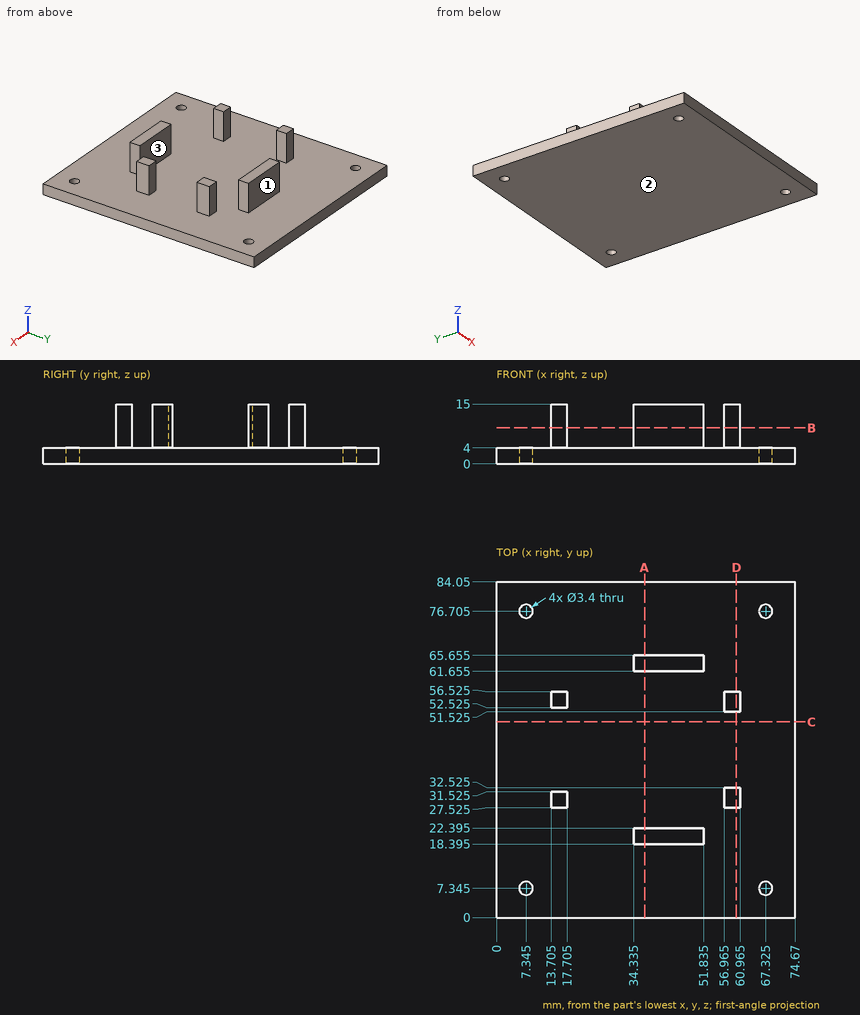
Geometry: see drawing. Coordinates: mm, zero at the bounding-box minimum. A direction names the side the tool comes from. Round coordinates to 2 decimals unless told otherwise and drop trailing zeros. Order: outer loops, then holes, each group sorted by start corner. A loop starts at its lowest first (then second) coordinate and runs counter-clockwise, first axis right, second up. Notation, with made-up numbers: (66.5, 57.25) -> (118.5, 57.25) arc R23 cw to (118.5, 86.25) -> close; hole circle Ø1 at (-29.5, 41). An arc over 180 degrees is marked (long way). Answer as CSV lines item,"result".
Item 1: Section A-A, the plane x = 37. Return loops of the section in (y, z) (3 decimals), plus the area to 3 significant figures.
A:
outline,"(0, 0) -> (84.05, 0) -> (84.05, 4) -> (65.655, 4) -> (65.655, 15) -> (61.655, 15) -> (61.655, 4) -> (22.395, 4) -> (22.395, 15) -> (18.395, 15) -> (18.395, 4) -> (0, 4) -> close"
area,"424 mm²"
Item 2: Reachability of the marked faces 1, 2 and 3 from +Z, -Z, +X, -X, +Y, -Y: full face, straight path, thin tool, end or side. Return the list, or none.
A:
face 1,"+Z, +X, -X, +Y"
face 2,"-Z, +X, -X, +Y, -Y"
face 3,"+Z, +X, -X"
Item 3: Pin query (flat end, axial travel): pin 1 Ø4.5 at (y, z) = (20.5, 10) entering from +X (3 decimals); pin 2 Ø3 at (x, z) = (15, 8.5) entering from -Y (3 decimals); pin 3 Ø3 at (x, z) = (50, 8.5) entering from -Y (3 decimals). Return the tip coordinate at first contact, or that it passes through.
A:
pin 1,"x = 51.835"
pin 2,"y = 27.525"
pin 3,"y = 18.395"
Item 4: Section D-D, the plane x = 60. Return loops of the section in (y, z) (3 decimals).
A:
outline,"(0, 0) -> (84.05, 0) -> (84.05, 4) -> (56.525, 4) -> (56.525, 15) -> (51.525, 15) -> (51.525, 4) -> (32.525, 4) -> (32.525, 15) -> (27.525, 15) -> (27.525, 4) -> (0, 4) -> close"
Item 5: Line query: L1, parallel to Y at x = 41, z = 10.5 (3 decimals); L2, parallel to Y at x = 59, z = 8 (3 decimals); L3, parallel to Z at x = 48, y = 79.5. Output: solid intervals per line, ascending.
A:
L1,"18.395 to 22.395, 61.655 to 65.655"
L2,"27.525 to 32.525, 51.525 to 56.525"
L3,"0 to 4"
Item 6: Section B-B, the plane z = 9. Return loops of the section in (x, y) (3 decimals).
A:
outline,"(13.705, 27.525) -> (17.705, 27.525) -> (17.705, 31.525) -> (13.705, 31.525) -> close; (13.705, 52.525) -> (17.705, 52.525) -> (17.705, 56.525) -> (13.705, 56.525) -> close; (34.335, 18.395) -> (51.835, 18.395) -> (51.835, 22.395) -> (34.335, 22.395) -> close; (34.335, 61.655) -> (51.835, 61.655) -> (51.835, 65.655) -> (34.335, 65.655) -> close; (56.965, 27.525) -> (60.965, 27.525) -> (60.965, 32.525) -> (56.965, 32.525) -> close; (56.965, 51.525) -> (60.965, 51.525) -> (60.965, 56.525) -> (56.965, 56.525) -> close"
Item 7: Section C-C, the plane y = 49. Return loops of the section in (x, z).
A:
outline,"(0, 0) -> (74.67, 0) -> (74.67, 4) -> (0, 4) -> close"
